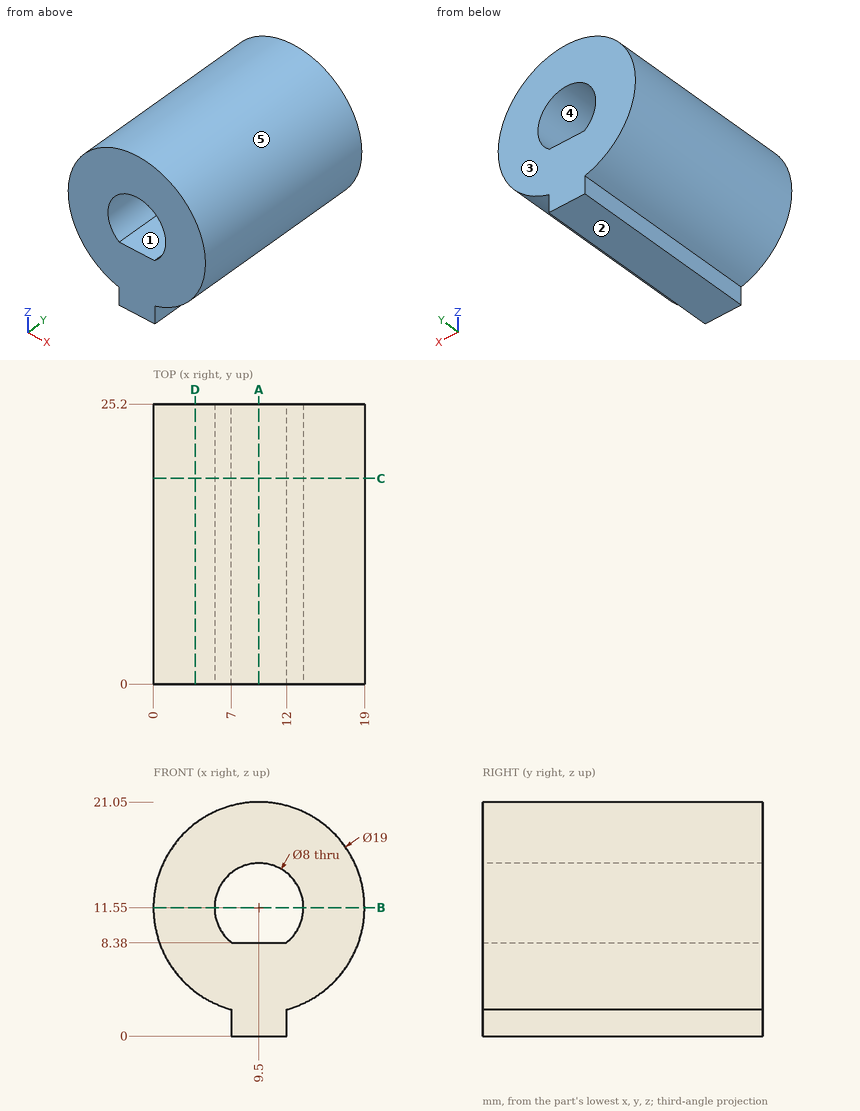
Here's the drawing with two shaded views (mm, measured from the low corner). I have some questions. A direction names the side the tool comes from. Give positions to 0.01 mm unless a question says otherwise; leave off trailing zeros. Loops run counter-clockwise (first coordinate to the right, second up) from the corner with the lowest first, then second, coordinate; pieces in that order, holes last. Notation, with made-up numbers: M 37,-27.75 L 90,-27.75 A19 cw 90,-21.75 Z; hole C -17,-35 d10. An arc over 180 degrees is marked long. One line per item, written item: value. Start each with the question number.
1) If we section it at B-B, the plane z = 11.55: Write out the boundary of the cut face in (x, y), and give its area (3 significant figures).
2) I'm going to push flat-ended pins straight in: pin 1 (6 mm diameter, centred on y = 6.5, z = 15, fed in from +X); pin 2 (10 mm diameter, centred on x = 15, y = 9.5, fed in from +Z); pin 3 (5 mm diameter, centred on x = 14, y = 15.5, fed in from +Z). Where does each tip first touch, or does it pass through?
3) If we section it at D-D, the plane x = 3.75: Write out the boundary of the cut face in (y, z).
4) If we section it at C-C, the plane y = 18.5: Write out the boundary of the cut face in (x, z), and give its area (3 significant figures).
5) On a 3-axis mill with a long thin cutter (end or side, diameter ignored), from which of +Z, -Z, +X, -X, +Y, -Y can I reach the whole of each face in a straight line? I mean the marked faces 1 and 2. Say none if no direction works.
6) If we section it at A-A, the plane x = 9.5: Write out the boundary of the cut face in (y, z), and give its area (3 significant figures).
7) Thinking about a two-plate mould opening in Z: for the marked faces 3, 4 and 5, which applies, +Z half, -Z half, draft (parallel to the pull), parting line (faces both ways), or undercut?
8) If I drill on line 1 (X direction, y = 16.75, z = 11.55); line 2 (X direction, y = 1.75, z = 8.25); line 3 (X direction, y = 12, z = 9), over which ranges is the centre line in solid material (lowest first)? Write a range as [from, to].
Completed:
1. outline: M 0,0 L 5.5,0 L 5.5,25.2 L 0,25.2 Z; M 13.5,0 L 19,0 L 19,25.2 L 13.5,25.2 Z
1. area: 277 mm^2
2. pin 1: stops at x = 18.99
2. pin 2: stops at z = 21.04
2. pin 3: stops at z = 20.84
3. outline: M 0,3.99 L 25.2,3.99 L 25.2,19.11 L 0,19.11 Z
4. outline: M 7,0 L 12,0 L 12,2.38 A9.5 ccw long 7,2.38 Z; hole M 7.06,8.38 L 11.94,8.38 A4 ccw long Z
4. area: 247 mm^2
5. face 1: +Y, -Y
5. face 2: -Z, +X, -X, +Y, -Y
6. outline: M 0,0 L 25.2,0 L 25.2,8.38 L 0,8.38 Z; M 0,15.55 L 25.2,15.55 L 25.2,21.05 L 0,21.05 Z
6. area: 350 mm^2
7. face 3: draft
7. face 4: undercut
7. face 5: parting line
8. line 1: x = [0, 5.5], [13.5, 19]
8. line 2: x = [0.59, 18.41]
8. line 3: x = [0.35, 6.42], [12.58, 18.65]
